```python
from build123d import *

# Parameters (mm, degrees)
SKETCH_1_R               = 4.95
SKETCH_1_R_2             = 3.5
EXTRUDE_1_DEPTH          = 37
CUT_EXTRUDE_START        = 11
SKETCH_1_3_R             = 4.95
SKETCH_1_3_R_2           = 3.5
CUT_EXTRUDE_1_DEPTH      = 2.6
CUT_EXTRUDE_START_2      = 19.7
SKETCH_1_4_R             = 4.95
SKETCH_1_4_R_2           = 3.5
CUT_EXTRUDE_2_DEPTH      = 2.6
SKETCH_2_R               = 1.5
CUT_EXTRUDE_3_DEPTH      = 10
SKETCH_3_R               = 1.6
CUT_EXTRUDE_4_DEPTH      = 38.656407157
CUT_EXTRUDE_START_3      = -7.3
SKETCH_4_R               = 4.95
SKETCH_4_R_2             = 4
CUT_EXTRUDE_5_DEPTH      = 1
CUT_EXTRUDE_START_4      = -25
SKETCH_4_2_R             = 4.95
SKETCH_4_2_R_2           = 4
CUT_EXTRUDE_6_DEPTH      = 1
CUT_EXTRUDE_7_DEPTH      = 38.656407184
CUT_EXTRUDE_7_DEPTH_BACK = 38.656407184
SKETCH_5_R               = 2


with BuildPart() as part:
    # Sketch 1 → Extrude 1 (new body)
    # profile 1 of 2: a face of its own
    with BuildSketch(Plane(origin=(0, 0, 0), x_dir=(0, 0, -1), z_dir=(1, 0, 0))):
        Circle(SKETCH_1_R)
        Circle(SKETCH_1_R_2, mode=Mode.SUBTRACT)
    # profile 2 of 2: a face of its own
    with BuildSketch(Plane(origin=(0, 0, 0), x_dir=(0, 0, -1), z_dir=(1, 0, 0))):
        Circle(SKETCH_1_R_2)
    extrude(amount=EXTRUDE_1_DEPTH)

    # Sketch 1_3 → Cut-Extrude 1 (cut)
    with BuildSketch(Plane(origin=(0, 0, 0), x_dir=(0, 0, -1), z_dir=(1, 0, 0)).offset(CUT_EXTRUDE_START)):
        Circle(SKETCH_1_3_R)
        Circle(SKETCH_1_3_R_2, mode=Mode.SUBTRACT)
    extrude(amount=CUT_EXTRUDE_1_DEPTH, mode=Mode.SUBTRACT)

    # Sketch 1_4 → Cut-Extrude 2 (cut)
    with BuildSketch(Plane(origin=(0, 0, 0), x_dir=(0, 0, -1), z_dir=(1, 0, 0)).offset(CUT_EXTRUDE_START_2)):
        Circle(SKETCH_1_4_R)
        Circle(SKETCH_1_4_R_2, mode=Mode.SUBTRACT)
    extrude(amount=CUT_EXTRUDE_2_DEPTH, mode=Mode.SUBTRACT)

    # Sketch 2 → Cut-Extrude 3 (cut)
    with BuildSketch(Plane.ZY):
        Circle(SKETCH_2_R)
    extrude(amount=-CUT_EXTRUDE_3_DEPTH, mode=Mode.SUBTRACT)

    # Sketch 3 → Cut-Extrude 4 (cut, through all)
    with BuildSketch(Plane(origin=(0, 0, 0), x_dir=(1, 0, 0), z_dir=(0, 1, 0))):
        with Locations(Location((3.3, 0, 0), (0, 0, 249.635865194))):
            Circle(SKETCH_3_R)
    extrude(amount=-CUT_EXTRUDE_4_DEPTH, mode=Mode.SUBTRACT)

    # Sketch 4 → Cut-Extrude 5 (cut)
    with BuildSketch(Plane.ZY.offset(CUT_EXTRUDE_START_3)):
        Circle(SKETCH_4_R)
        Circle(SKETCH_4_R_2, mode=Mode.SUBTRACT)
    extrude(amount=-CUT_EXTRUDE_5_DEPTH, mode=Mode.SUBTRACT)

    # Sketch 4_2 → Cut-Extrude 6 (cut)
    with BuildSketch(Plane.ZY.offset(CUT_EXTRUDE_START_4)):
        Circle(SKETCH_4_2_R)
        Circle(SKETCH_4_2_R_2, mode=Mode.SUBTRACT)
    extrude(amount=-CUT_EXTRUDE_6_DEPTH, mode=Mode.SUBTRACT)

    # Sketch 5 → Cut-Extrude 7 (cut, two sides: drawn at the far end of the back side and taken through both)
    with BuildSketch(Plane(origin=(0, 0, 0), x_dir=(1, 0, 0), z_dir=(0, 1, 0)).offset(-CUT_EXTRUDE_7_DEPTH_BACK)):
        with Locations(Location((32, 0, 0), (0, 0, 270))):
            Circle(SKETCH_5_R)
    extrude(amount=CUT_EXTRUDE_7_DEPTH + CUT_EXTRUDE_7_DEPTH_BACK, mode=Mode.SUBTRACT)


solid = part.part
```
Can you work these out from the model? Positions are in its coordinate system, mm. A direction names the side the tool comes from. Give positions to 0.01 mm unless a question says otherwise; leave off trailing zeros. Loops run counter-clockwise (first coordinate to the right, second up) from the corner with the lowest first, then second, coordinate; pieces in that order, holes last. Notation, with made-up numbers: M -32,18 L 16,18 A15 ccw 16,29 Z; hole C 86,51 d7. An arc over 180 degrees is marked long. One line per question, with ' | ' between items. Start each with the question number.
Q1. If we mould it in two halves opening along Z, with no side actions, what happens to faces 1 (the cylindrical face through (4.93, 1.487, -0.195)), 2 (the cylindrical face through (3.599, 4.174, -2.661)), 3 (the flat face through (11, -3.2, -2.1))? For each: +Z half, -Z half, draft (parallel to the pull), parting line (faces both ways), or undercut.
Q2. For pin 1 Ø1 at (x, y) = (26.5, -3) entering from +Z; pin 2 Ø0.9 at (y, z) = (0, 0.5) entering from -X; pin 3 Ø5 at (x, y) = (26.5, 3.5) entering from -Z, each with a flat end and sliding along its axis, tell me the tip position at first contact or that it passes through.
Q3. If I drill on line 1 (X direction, y = 4.75, z = 0); line 2 (X direction, y = -2.15, z = 0); line 3 (X direction, y = -2, z = -0.75), over which ranges is the centre line in solid material (lowest first)? Write a range as from..to.
Q4. If we section it at A-A (z = 0): State how many separate pieces and enclosed holes the cut face has, plus the area to 3 significant figures.
Q5. If we section it at B-B (x = 31): Please give me the cut outline in (y, z).
Q6. If we section it at D-D (x = 3.3): Please give me the cut outline in (y, z), plus the area to 3 significant figures.
Q7. For faces 4 (the flat face through (8.3, -4, 2)), 5 (the flat face through (10, 0, 0)), 6 (the cylindrical face through (23.63, 1.49, -4.72)), which set-ups out of +Z, -Z, +X, -X, +Y, -Y let a thin tool reach every point of the face, with its end or its side?
Computed:
1) face 1: undercut | face 2: parting line | face 3: draft
2) pin 1: stops at z = 4.27 | pin 2: stops at x = 10 | pin 3: stops at z = -4.85
3) line 1: x = 0..7.3, 8.3..11, 13.6..19.7, 22.3..25, 26..30, 34..37 | line 2: x = 0..1.7, 4.9..30, 34..37 | line 3: x = 0..1.89, 4.71..30.15, 33.85..37
4) separate pieces: 3 | enclosed holes: 0 | area: 267 mm²
5) outline: M -4.64,-1.73 A4.95 ccw 4.64,-1.73 Z; M -4.64,1.73 L 4.64,1.73 A4.95 ccw Z
6) outline: M -4.68,-1.6 A4.95 ccw long -4.68,1.6 L 0,1.6 L 0,1.5 A1.5 cw 0,-1.5 L 0,-1.6 Z | area: 57.9 mm²
7) face 4: none | face 5: -X | face 6: +X, -X
